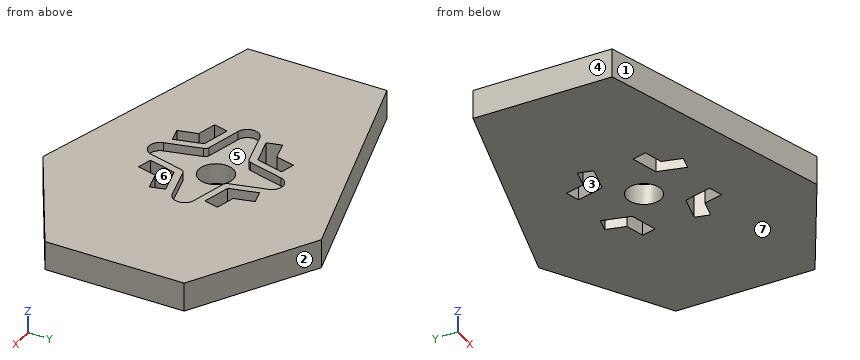
from build123d import *

# Parameters (mm, degrees)
SKETCH1_R            = 3.45
BOSS_EXTRUDE1_DEPTH  = 4.1
BOSS_EXTRUDE2_DEPTH  = 5.8
CUT_EXTRUDE1_DEPTH   = 51.416317693
MIRROR2_COPY_1_DEPTH = 51.416317693


with BuildPart() as part:
    # Sketch1 → Boss-Extrude1 (new body)
    with BuildSketch(Plane.XY):
        Polygon((6.974355653, -28), (-41.523066959, -14), (-41.523066959, 14), (6.974355653, 28), (31.223066959, 14), (31.223066959, -14), align=None)
        with Locations((-5.15, 0)):
            Circle(SKETCH1_R, mode=Mode.SUBTRACT)
    extrude(amount=BOSS_EXTRUDE1_DEPTH)

    # Sketch1<3> → Boss-Extrude2 (add)
    with BuildSketch(Plane.XY):
        Polygon((-41.523066959, -14), (6.974355653, -28), (31.223066959, -14), (31.223066959, 14), (6.974355653, 28), (-41.523066959, 14), align=None)
        with BuildLine():
            Line((-1.14034217, -4.727614303), (-2.971580528, -11.813017409))
            ThreePointArc((-2.971580528, -11.813017409), (-5.15, -13.5), (-7.328419472, -11.813017409))
            Line((-7.328419472, -11.813017409), (-9.15965783, -4.727614303))
            ThreePointArc((-9.15965783, -4.727614303), (-9.420737481, -4.270737481), (-9.877614303, -4.00965783))
            Line((-9.877614303, -4.00965783), (-16.963017409, -2.178419472))
            ThreePointArc((-16.963017409, -2.178419472), (-18.65, 0), (-16.963017409, 2.178419472))
            Line((-16.963017409, 2.178419472), (-9.877614303, 4.00965783))
            ThreePointArc((-9.877614303, 4.00965783), (-9.420737481, 4.270737481), (-9.15965783, 4.727614303))
            Line((-9.15965783, 4.727614303), (-7.328419472, 11.813017409))
            ThreePointArc((-7.328419472, 11.813017409), (-5.15, 13.5), (-2.971580528, 11.813017409))
            Line((-2.971580528, 11.813017409), (-1.14034217, 4.727614303))
            ThreePointArc((-1.14034217, 4.727614303), (-0.879262519, 4.270737481), (-0.422385697, 4.00965783))
            Line((-0.422385697, 4.00965783), (6.663017409, 2.178419472))
            ThreePointArc((6.663017409, 2.178419472), (8.35, 0), (6.663017409, -2.178419472))
            Line((6.663017409, -2.178419472), (-0.422385697, -4.00965783))
            ThreePointArc((-0.422385697, -4.00965783), (-0.879262519, -4.270737481), (-1.14034217, -4.727614303))
        make_face(mode=Mode.SUBTRACT)
    extrude(amount=BOSS_EXTRUDE2_DEPTH)

    # Sketch3 → Cut-Extrude1 (cut, through all)
    with BuildSketch(Plane.XY.offset(5.8)):
        Polygon((-13.000425446, 7.850425446), (-16.873171174, 6.849505608), (-16.122481296, 3.944946311), (-10.538213003, 5.388213003), (-9.094946311, 10.972481296), (-11.999505608, 11.723171174), align=None)
    cut_extrude1 = extrude(amount=-CUT_EXTRUDE1_DEPTH, mode=Mode.SUBTRACT)

    # Mirror1: Cut-Extrude1 across plane
    add(cut_extrude1.mirror(Plane.ZY.offset(5.15)), mode=Mode.SUBTRACT)

    # Mirror2: Cut-Extrude1 across plane
    add(cut_extrude1.mirror(Plane(origin=(0, 0, 0), x_dir=(0, 0, 1), z_dir=(0, -1, 0))), mode=Mode.SUBTRACT)

    # Mirror2 copy 1 sketch → Mirror2 copy 1 (cut, through all)
    with BuildSketch(Plane(origin=(-10.3, 0, 5.8), x_dir=(-1, 0, 0), z_dir=(0, 0, 1))):
        Polygon((-13.000425446, 7.850425446), (-16.873171174, 6.849505608), (-16.122481296, 3.944946311), (-10.538213003, 5.388213003), (-9.094946311, 10.972481296), (-11.999505608, 11.723171174), align=None)
    extrude(amount=-MIRROR2_COPY_1_DEPTH, mode=Mode.SUBTRACT)


solid = part.part
The listing builds one solid part. Answer for the finished solid, in the listing's coordinates (mm). Face numbers are marked on the shaded views. A direction names the side the tool comes from. Round coordinates to 2 decimals unless told otherwise and drop trailing zeros. Write each loop counter-clockwise with the first axis right and the second up, starting at its lowest first coordinate (ties: lowest second). Pieces come first, ordered by that corner, then holes. Notation, with made-up numbers: (68, -34.75) - (93, -34.75) arc R19 cw to (93, 2.25) - close; hole circle Ø4 at (13.25, 35). An arc over 180 degrees is marked (long way). Use one line per item in the form item = value. Start each with the question number.
Item 1: Flat-ended cylindrical pins translate along their axes: pin 1 Ø2 at (x, z) = (-0.5, 4) entering from +Y; pin 2 Ø21.5 at (x, y) = (-6, -2.5) entering from +Z; pin 3 Ø1 at (y, z) = (-22, 4.5) entering from +X; pin 4 Ø2 at (x, z) = (-28, 5) entering from -Y. Find the tip coordinate at first contact, or state that the pin passes through.
Item 2: A cutting plane is placed at D-D (x = 5). Write down the section's boundary in (y, z), plus the area to 3 significant figures.
Item 3: A cutting plane is placed at C-C (z = 0.75). Give the number of separate pieces and of enclosed holes in the cut face, plus the area to 3 significant figures.
Item 4: A cutting plane is placed at B-B (y = 0). Write down the section's boundary in (x, z), plus the area to 3 significant figures.
Item 5: Determine the mould class of the marked faces 1, 2, 3 and 4 for opening direction Y: +Y half, -Y half, draft (parallel to the pull), parting line (faces both ways), or undercut.
Item 6: A cutting plane is placed at A-A (x = -5.15). Write down the section's boundary in (y, z).
Item 7: A tool of negligible diameter and unlimited length cuts with its end or side. For the marked faces 5, 6 and 7, from which of +Z, -Z, +X, -X, +Y, -Y can it reach the whole face along a straight path? Write none if from no direction.
Item 8: Find the intervals of material crossed by line 1 (Y direction, x = -5.15, z = 3.05); line 2 (X direction, y = 0.5, z = 3.2); line 3 (Y direction, x = 0.5, z = 4.2), in increasing order. Write a range as [from, to].
The answers:
q1.pin_1 = 26.13
q1.pin_2 = 5.8
q1.pin_3 = 18.23
q1.pin_4 = -18.19
q2.outline = (-27.43, 0) - (-7.26, 0) - (-7.26, 5.8) - (-27.43, 5.8) - close; (-4.16, 0) - (4.16, 0) - (4.16, 5.8) - (2.61, 5.8) - (2.61, 4.1) - (-2.61, 4.1) - (-2.61, 5.8) - (-4.16, 5.8) - close; (7.26, 0) - (27.43, 0) - (27.43, 5.8) - (7.26, 5.8) - close
q2.area = 273 mm^2
q3.separate_pieces = 1
q3.enclosed_holes = 5
q3.area = 2,900 mm^2
q4.outline = (-41.52, 0) - (-8.6, 0) - (-8.6, 4.1) - (-18.65, 4.1) - (-18.65, 5.8) - (-41.52, 5.8) - close; (-1.7, 0) - (31.22, 0) - (31.22, 5.8) - (8.35, 5.8) - (8.35, 4.1) - (-1.7, 4.1) - close
q4.area = 348 mm^2
q5.face_1 = -Y half
q5.face_2 = +Y half
q5.face_3 = undercut
q5.face_4 = draft
q6.outline = (-24.5, 0) - (-3.45, 0) - (-3.45, 4.1) - (-13.5, 4.1) - (-13.5, 5.8) - (-24.5, 5.8) - close; (3.45, 0) - (24.5, 0) - (24.5, 5.8) - (13.5, 5.8) - (13.5, 4.1) - (3.45, 4.1) - close
q7.face_5 = +Z
q7.face_6 = +Z, -Z
q7.face_7 = -Z, +X, -X, +Y, -Y
q8.line_1 = [-24.5, -3.45], [3.45, 24.5]
q8.line_2 = [-41.52, -8.56], [-1.74, 31.22]
q8.line_3 = [-26.13, -11.41], [-5.32, -3.77], [3.77, 5.32], [11.41, 26.13]
